The drawing under review shows one solid part. Ordinate dimensions are in mm from its lowest x, y, z. A direction names the side the tool comes from. Give positions to 0.01 mm unless a question says otherwise; leave off trailing zeros. Order: outer loops, then holes, each group sorted by start corner. A loop starts at its lowest first (then second) coordinate and runs counter-clockwise, first axis right, second up. Notation, with made-up numbers: (-6, -29) -> (52, -29) arc R25 ccw to (52, -17) -> close; hole circle Ø4 at (-38.5, 6.5). An arc over 180 degrees is marked (long way). Return JSON: item names as keys, results as strings. Group by question number.
1) Insertion check: P1, Ø15.5, axis at x = 30.5, y = 39, coming from the +Z side; P2, Ø6, axis at x = 47.625, z = 6.35, coming from the +Y side. Each pin has a flat end and moves straight along its axis. Give the tip position at first contact, or say it passes through.
2) Add section B-B (y = 9). Give the boundary of the cut face in (x, z) (3 decimals), then the cut area to 3 significant figures.
3) Add section D-D (y = 41). State how many separate pieces and enclosed holes the cut face has, then the cut area to 3 significant figures.
4) For the marked faces 1, 2 and 3, list the 3-axis set-ups (+Z, -Z, +X, -X, +Y, -Y) from which the entire face can be reached by the end or side of a thin tool; tool diameter is ignored.
5) To check wall thickness, follow line 1 along X through (y, z) = (53, 5.5) (1 decimal); line 2 along X through (y, z) = (29.5, 7.5) (1 decimal); line 3 along X through (y, z) = (24, 4.25). State the ranges of each line that lie inside material, in increasing order.
6) The part is to be moulded in two halves that separate along Z. For the marked faces 4, 5 and 6, say which applies: released by +Z, released by -Z, zero draft, split by the parting line, or undercut.
7) Add section A-A (x = 31.75). Give the boundary of the cut face in (y, z).
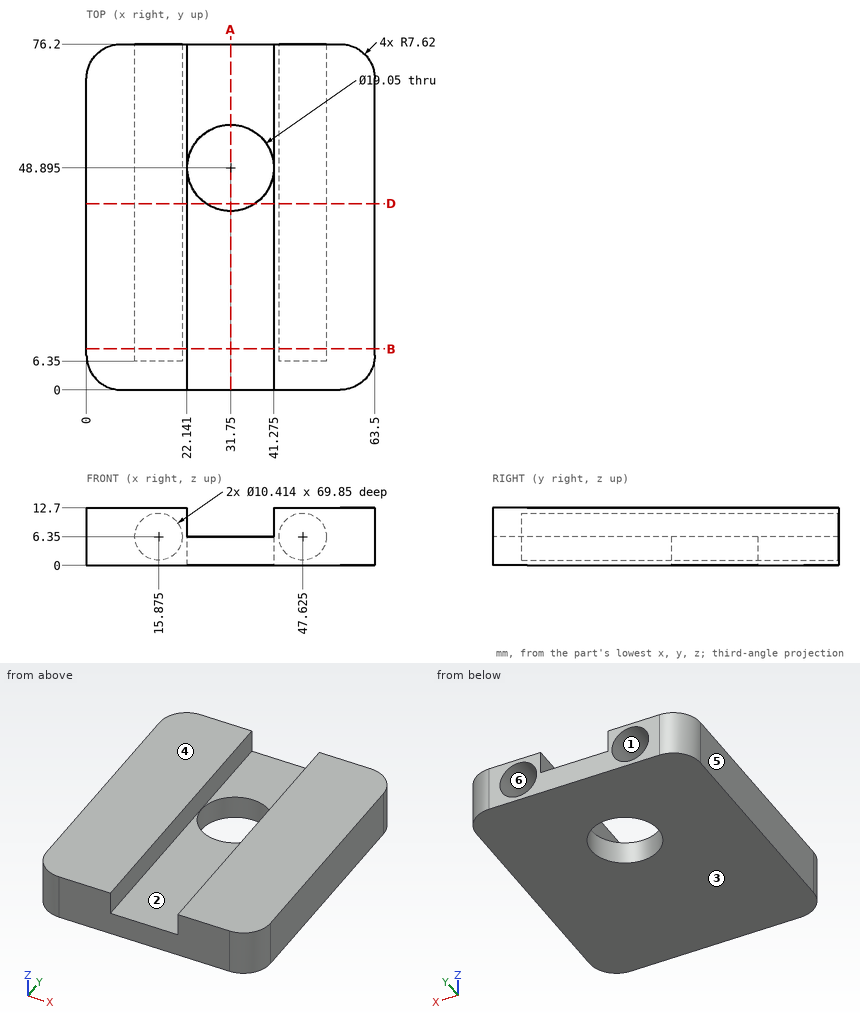
Evaluation:
{
 "1": {"P1": "z = 6.35", "P2": "y = 6.35"},
 "2": {"outline": "(0, 0) -> (63.5, 0) -> (63.5, 12.7) -> (41.275, 12.7) -> (41.275, 6.35) -> (22.141, 6.35) -> (22.141, 12.7) -> (0, 12.7) -> close; hole circle Ø10.414 at (15.875, 6.35); hole circle Ø10.414 at (47.625, 6.35)", "area": "515 mm^2"},
 "3": {"separate pieces": "2", "enclosed holes": "2", "area": "447 mm^2"},
 "4": {"face 1": "+Y", "face 2": "+Z, +Y, -Y", "face 3": "-Z, +X, -X, +Y, -Y"},
 "5": {"line 1": "0 to 10.7, 21 to 23.2, 40.3 to 42.5, 52.8 to 63.5", "line 2": "0 to 10.8, 21 to 22.1, 41.3 to 42.5, 52.7 to 63.5", "line 3": "0 to 11.11, 20.64 to 42.86, 52.39 to 63.5"},
 "6": {"face 4": "released by +Z", "face 5": "zero draft", "face 6": "undercut"},
 "7": {"outline": "(0, 0) -> (39.37, 0) -> (39.37, 6.35) -> (0, 6.35) -> close; (58.42, 0) -> (76.2, 0) -> (76.2, 6.35) -> (58.42, 6.35) -> close"}
}
